Verification items for the finished model (mm, model axes). A direction names the side the tool comes from. Round coordinates to 2 decimals unless told otherwise and drop trailing zeros. Write each loop counter-clockwise with the first axis right and the second up, starting at its lowest first coordinate (ties: lowest second). Pieces come first, ordered by that corner, then holes. Notation, with made-up numbers: (27, 87.25) - (83, 87.25) arc R21 ccw to (83, 125.25) - close; hole circle Ø8 at (49, 3.25). An arc over 180 degrees is marked (long way). Answer as a JSON object with one key per item and string values.
```python
from build123d import *

# Parameters (mm, degrees)
SKETCH_1_R          = 5
EXTRUDE_1_DEPTH     = 5
SKETCH_2_R          = 10
SKETCH_2_R_2        = 5
EXTRUDE_2_DEPTH     = 33.2
SKETCH_4_R          = 16
CUT_EXTRUDE_2_DEPTH = 15
SKETCH_7_R          = 19
SKETCH_7_R_2        = 16
EXTRUDE_3_DEPTH     = 7
SKETCH_8_R          = 19
SKETCH_8_R_2        = 7.5
EXTRUDE_4_DEPTH     = 2
CUT_EXTRUDE_3_DEPTH = 10
SKETCH_10_R         = 2
CUT_EXTRUDE_4_DEPTH = 10


with BuildPart() as part:
    # 草图1 → 凸台-拉伸1 (new body)
    with BuildSketch(Plane.XY):
        with BuildLine():
            ThreePointArc((-128.022678922, -73.913928138), (-90.421378279, 38.440519474), (0, 115))
            ThreePointArc((0, 115), (90.421378279, 38.440519474), (128.022678922, -73.913928138))
            ThreePointArc((128.022678922, -73.913928138), (0, -115), (-128.022678922, -73.913928138))
        make_face()
        with Locations((0, 103)):
            Circle(SKETCH_1_R, mode=Mode.SUBTRACT)
        with Locations((-117.630374076, -67.913928138)):
            Circle(SKETCH_1_R, mode=Mode.SUBTRACT)
        with Locations((117.630374076, -67.913928138)):
            Circle(SKETCH_1_R, mode=Mode.SUBTRACT)
    extrude(amount=EXTRUDE_1_DEPTH)

    # 草图2 → 凸台-拉伸2 (add)
    # profile 1 of 3: a face of its own
    with BuildSketch(Plane.XY.offset(5)):
        with Locations(Location((0, 103, 0), (0, 0, 180))):
            Circle(SKETCH_2_R)
        with Locations((0, 103)):
            Circle(SKETCH_2_R_2, mode=Mode.SUBTRACT)
    # profile 2 of 3: a face of its own
    with BuildSketch(Plane.XY.offset(5)):
        with Locations(Location((-117.630374076, -67.913928138, 0), (0, 0, 179.375778052))):
            Circle(SKETCH_2_R)
        with Locations((-117.630374076, -67.913928138)):
            Circle(SKETCH_2_R_2, mode=Mode.SUBTRACT)
    # profile 3 of 3: a face of its own
    with BuildSketch(Plane.XY.offset(5)):
        with Locations(Location((117.630374076, -67.913928138, 0), (0, 0, 8.696571879))):
            Circle(SKETCH_2_R)
        with Locations((117.630374076, -67.913928138)):
            Circle(SKETCH_2_R_2, mode=Mode.SUBTRACT)
    extrude(amount=EXTRUDE_2_DEPTH)

    # 草图4 → 切除-拉伸2 (cut)
    with BuildSketch(Plane(origin=(0, 0, 0), x_dir=(-1, 0, 0), z_dir=(0, 0, -1))):
        with Locations((-12.650995066, 69.515536741)):
            Circle(SKETCH_4_R)
        with Locations((-82.334125615, -39.530718783)):
            Circle(SKETCH_4_R)
    extrude(amount=-CUT_EXTRUDE_2_DEPTH, mode=Mode.SUBTRACT)

    # 草图7 → 凸台-拉伸3 (add)
    # profile 1 of 2: a face of its own
    with BuildSketch(Plane.XY.offset(5)):
        with Locations((82.334125615, -39.530718783)):
            Circle(SKETCH_7_R)
        with Locations(Location((82.334125615, -39.530718783, 0), (0, 0, 180))):
            Circle(SKETCH_7_R_2, mode=Mode.SUBTRACT)
    # profile 2 of 2: a face of its own
    with BuildSketch(Plane.XY.offset(5)):
        with Locations((12.650995066, 69.515536741)):
            Circle(SKETCH_7_R)
        with Locations(Location((12.650995066, 69.515536741, 0), (0, 0, 180))):
            Circle(SKETCH_7_R_2, mode=Mode.SUBTRACT)
    extrude(amount=EXTRUDE_3_DEPTH)

    # 草图8 → 凸台-拉伸4 (add)
    # profile 1 of 2: a face of its own
    with BuildSketch(Plane.XY.offset(12)):
        with Locations((82.334125615, -39.530718783)):
            Circle(SKETCH_8_R)
        with Locations((82.334125615, -39.530718783)):
            Circle(SKETCH_8_R_2, mode=Mode.SUBTRACT)
    # profile 2 of 2: a face of its own
    with BuildSketch(Plane.XY.offset(12)):
        with Locations((12.650995066, 69.515536741)):
            Circle(SKETCH_8_R)
        with Locations((12.650995066, 69.515536741)):
            Circle(SKETCH_8_R_2, mode=Mode.SUBTRACT)
    extrude(amount=EXTRUDE_4_DEPTH)

    # 草图9 → 切除-拉伸3 (cut)
    with BuildSketch(Plane(origin=(0, 0, 0), x_dir=(-1, 0, 0), z_dir=(0, 0, -1))):
        Polygon((20.065498734, -11.479666127), (28.668863324, -50.543487212), (9.136952782, -54.845169507), (0.533588192, -15.781348422), align=None)
    extrude(amount=-CUT_EXTRUDE_3_DEPTH, mode=Mode.SUBTRACT)

    # 草图10 → 切除-拉伸4 (cut)
    with BuildSketch(Plane.XY.offset(5)):
        with Locations((-24.807535234, -56.257736539)):
            Circle(SKETCH_10_R)
        with Locations((-15.041579962, -58.408577687)):
            Circle(SKETCH_10_R)
        with Locations((-14.160871553, -7.916257947)):
            Circle(SKETCH_10_R)
        with Locations((-4.394916282, -10.067099095)):
            Circle(SKETCH_10_R)
    extrude(amount=-CUT_EXTRUDE_4_DEPTH, mode=Mode.SUBTRACT)


solid = part.part
```
Q1. Set-up check for faces 5 (the flat face through (12, 61, 14)), 6 (the flat face through (-24.3, -30.7, 2.5)), 7 (the cylindrical face through (100.457, -33.824, 9.437)): record each of +Z, -Z, +X, -X, +Y, -Y from which the full face is reachable in a straight line by a thin tool's end or side.
Geometry check:
{"face 5": "+Z, +X, -X, -Y", "face 6": "+Z, -Z", "face 7": "+Z"}
Q2. Material ranges on line 1 along Z through (x, y) = (67.5, -93); line 2 along Y through (x, z) = (14, 6); line 3 along Y through (x, z) = (93.5, 7), recorded low to high. Write a range as [from, to].
Geometry check:
{"line 1": "z = [0, 5]", "line 2": "y = [50.56, 53.57], [85.46, 88.47]", "line 3": "y = [-54.9, -50.99], [-28.07, -24.16]"}
Q3. Release check for a two-part mould opening along X. For faces 1 (the flat face through (113, -71, 38.2)), 2 (the cylindrical face through (74.84, -39.2, 12.99)), 3 (the cylindrical face through (1.91, -114.99, 2.46)), 4 (the flat face through (-4.9, -35.6, 2.5)) record: released by +X, released by -X, zero draft, split by the parting line, or undercut.
Geometry check:
{"face 1": "zero draft", "face 2": "undercut", "face 3": "split by the parting line", "face 4": "undercut"}
Q4. Section check A-A, the plane z = 26. Record the cut outline in (x, y), then the cut area to 3 significant figures.
Geometry check:
{"outline": "circle Ø20 at (-117.63, -67.91); circle Ø20 at (0, 103); circle Ø20 at (117.63, -67.91); hole circle Ø10 at (-117.63, -67.91); hole circle Ø10 at (0, 103); hole circle Ø10 at (117.63, -67.91)", "area": "707 mm2"}
Q5. Section check D-D, the plane y = -87.5. Record the cut outline in (x, z).
Geometry check:
{"outline": "(-106.51, 0) - (106.51, 0) - (106.51, 5) - (-106.51, 5) - close"}
Q6. Gauge pin test, flat ends, axial feed: P1, Ø3.5, axis at x = -15.04, y = -58.41, coming from the -Z side; P2, Ø8, axis at y = -67, z = 31, coming from the +X side; P3, Ø19, axis at x = 78.5, y = -39, coming from the +Z side; P4, Ø5, axis at x = 95.5, y = 20.5, coming from the +Z side. Record the tip position at first contact, or that the pin passes through.
Geometry check:
{"P1": "passes through", "P2": "stops at x = 127.63", "P3": "stops at z = 14", "P4": "stops at z = 5"}
Q7. Section check B-B, the plane y = 81. Record the cut outline in (x, z).
Geometry check:
{"outline": "(-52.7, 0) - (1.51, 0) - (1.51, 12) - (23.79, 12) - (23.79, 0) - (52.7, 0) - (52.7, 5) - (27.79, 5) - (27.79, 14) - (-2.49, 14) - (-2.49, 5) - (-52.7, 5) - close"}
Q8. Section check C-C, the plane y = 38.5. Record the cut outline in (x, z).
Geometry check:
{"outline": "(-90.38, 0) - (90.38, 0) - (90.38, 5) - (-90.38, 5) - close"}
